Geometry: final body of the model. Coordinates: model frame, mm. A direction names the side the tool comes from. Round coordinates to 2 decimals unless told otherwise and drop trailing zeros. Order: outer loops, then holes, each group sorted by start corner. A loop starts at its lowest first (then second) coordinate and runs counter-clockwise, first axis right, second up. Notation, with made-up numbers: (66.25, 88) - (100.25, 88) arc R17 ccw to (100.25, 108) - close; hole circle Ø2 at (-29.5, -31.75). An arc over 180 degrees is marked (long way). Put each result on its own line as item: value. Start each with the question number.
(1) Material intervals for L1, parallel to Y at x = 111, z = 215; L2, parallel to X at y = -8.5, z = 230; L3, parallel to Z at x = -26, y = 73, sorted ascending. Write a range as [from, to].
(2) Section C-C (z = 185). Output: boundary loops of the cut face in (x, y), and give its area (3 significant figures).
(3) Pull-direction query (Y, two-part tool) for faces 1 (the face through (165.1, -3, 138)), 2 (the face through (-2, -190.5, 138)), 3 (the face through (-2, 187.96, 139)), 4 (the face through (-2, 190.5, 138)); classes: released by +Y, released by -Y, zero draft, split by the parting line, or undercut.
(4) Section B-B (x = -37). Output: boundary loops of the cut face in (y, z), and give its area (3 significant figures).
(5) Pin query (flat end, axial travel): P1, Ø8, axis at x = -130.5, y = -136.5, coming from the +Z side. Return the tip coordinate at first contact, or that it passes through.
(6) Section A-A (z = 228). Output: boundary loops of the cut face in (x, y), and give its area (3 significant figures).
(7) Access query for faces 5 (the face through (-2, 3, 2.54)), 6 (the face through (-2, 3, 0)). Directions: +Z, -Z, +X, -X, +Y, -Y. A direction counts if a zero-diameter tool reaches every point of the face in a straight line with its end or side. Return the directions, or none.
(8) Section D-D (x = 69). Output: boundary loops of the cut face in (y, z), and give its area (3 significant figures).
from build123d import *

# Parameters (mm, degrees)
F0_W     = 330.2
F0_H     = 381
F1_DEPTH = 279.4
F2_T     = -2.54
F3_W     = 127
F3_H     = 25.4
F4_DEPTH = 381.001


with BuildPart() as f1:
    # F0 (on Top) → F1 (new body)
    with BuildSketch(Plane.XY):
        Rectangle(F0_W, F0_H)
    extrude(amount=F1_DEPTH)

    # F2
    f2_openings = [f1.faces().sort_by_distance(p)[0] for p in [
        (0, 0, 279.4),
    ]]
    offset(amount=F2_T, openings=f2_openings)

    # F3 (on face) → F4 (cut, through all)
    with BuildSketch(Plane.XZ.offset(190.5)):
        with Locations((0, 228.6)):
            Rectangle(F3_W, F3_H)
    extrude(amount=-F4_DEPTH, mode=Mode.SUBTRACT)


solid = f1.part
Checks:
1. L1: y = [-190.5, -187.96], [187.96, 190.5]
1. L2: x = [-165.1, -162.56], [162.56, 165.1]
1. L3: z = [0, 2.54]
2. outline: (-165.1, -190.5) - (165.1, -190.5) - (165.1, 190.5) - (-165.1, 190.5) - close; hole (-162.56, -187.96) - (162.56, -187.96) - (162.56, 187.96) - (-162.56, 187.96) - close
2. area: 3,590 mm²
3. face 1: zero draft
3. face 2: released by -Y
3. face 3: undercut
3. face 4: released by +Y
4. outline: (-190.5, 0) - (190.5, 0) - (190.5, 215.9) - (187.96, 215.9) - (187.96, 2.54) - (-187.96, 2.54) - (-187.96, 215.9) - (-190.5, 215.9) - close; (-190.5, 241.3) - (-187.96, 241.3) - (-187.96, 279.4) - (-190.5, 279.4) - close; (187.96, 241.3) - (190.5, 241.3) - (190.5, 279.4) - (187.96, 279.4) - close
4. area: 2,250 mm²
5. P1: stops at z = 2.54
6. outline: (-165.1, -190.5) - (-63.5, -190.5) - (-63.5, -187.96) - (-162.56, -187.96) - (-162.56, 187.96) - (-63.5, 187.96) - (-63.5, 190.5) - (-165.1, 190.5) - close; (63.5, -190.5) - (165.1, -190.5) - (165.1, 190.5) - (63.5, 190.5) - (63.5, 187.96) - (162.56, 187.96) - (162.56, -187.96) - (63.5, -187.96) - close
6. area: 2,940 mm²
7. face 5: +Z
7. face 6: -Z, +X, -X, +Y, -Y
8. outline: (-190.5, 0) - (190.5, 0) - (190.5, 279.4) - (187.96, 279.4) - (187.96, 2.54) - (-187.96, 2.54) - (-187.96, 279.4) - (-190.5, 279.4) - close
8. area: 2,370 mm²
